Autodesk Inventor part; units mm, degrees
ref_plane "YZ Plane" through (0, 0, 0) normal (1, 0, 0) x (0, 1, 0)
ref_plane "XZ Plane" through (0, 0, 0) normal (0, 1, 0) x (-1, 0, 0)
ref_plane "XY Plane" through (0, 0, 0) normal (0, 0, 1) x (1, 0, 0)
sketch "Sketch1" plane through (0, 0, 0) normal (0, 0, 1) x (1, 0, 0)
  line L0 (0, 0) -> (3294.2276, 1099.144)
  line L1 (3294.2276, 1246.4151) -> (-135.0962, 102.1952)
  line L2 (0, 0) -> (-135.0962, 0)
  line L3 (-135.0962, 0) -> (-135.0962, 102.1952)
  line L4 (-135.0962, 102.1952) -> (1627.6312, 690.3426)
  line L5 (3294.2276, 1099.144) -> (3263.9, 1099.144)
  line L6 (3294.2276, 1099.144) -> (3294.2276, 1246.4151)
  line L7 (-88.9, 0) -> (-88.9, 117.6089)
  line L8 (3263.9, 1089.025) -> (3263.9, 1236.2961)
  line L9 (-135.0962, 102.1952) -> (-160.4962, 102.1952)
  line L10 (-160.4962, 102.1952) -> (-160.4962, 0)
  line L11 (-160.4962, 0) -> (-135.0962, 0)
  line L12 (-135.0962, 102.1952) -> (-140.1208, 117.2541)
  line L13 (-140.1208, 117.2541) -> (150.6173, 214.261)
  line L14 (150.6173, 214.261) -> (155.6418, 199.2021)
  line L15 (-27.6261, 154.7888) -> (-28.631, 157.8005)
  line L16 (-28.631, 157.8005) -> (-173.1962, 109.5652)
  line L17 (-173.1962, 109.5652) -> (-163.6712, 101.107)
  line L18 (-163.6712, 101.107) -> (-163.6712, 92.6488)
  line L19 (-163.6712, 92.6488) -> (-173.1962, 86.9102)
  line L20 (-171.5578, 84.1906) -> (-160.4962, 90.855)
  line L21 (-160.4962, 90.855) -> (-160.4962, 102.5338)
  line L22 (-160.4962, 102.5338) -> (-166.9808, 108.292)
  line L23 (-166.9808, 108.292) -> (-27.6261, 154.7888)
  line L24 (-171.5578, 84.1906) -> (-173.1962, 86.9102)
  line L25 (-173.1962, 109.5652) -> (-173.1962, 86.9102)
  line L26 (3163.3672, 1202.7525) -> (3162.3623, 1205.7643)
  line L27 (3162.3623, 1205.7643) -> (3306.9276, 1253.9996)
  line L28 (3163.3672, 1202.7525) -> (3293.697, 1246.2381)
  line L29 (3293.697, 1246.2381) -> (3294.2276, 1246.7092)
  line L30 (3306.9276, 1253.9996) -> (3297.4026, 1245.5414)
  line L31 (3297.4026, 1245.5414) -> (3297.4026, 1237.0832)
  line L32 (3294.2276, 1246.7092) -> (3294.2276, 1235.2894)
  line L33 (3297.4026, 1237.0832) -> (3306.9276, 1231.3446)
  line L34 (3306.9276, 1231.3446) -> (3305.2891, 1228.625)
  line L35 (3305.2891, 1228.625) -> (3294.2276, 1235.2894)
  line L36 (3306.9276, 1253.9996) -> (3306.9276, 1231.3446)
  point P0 (-160.4962, 90.855)
  point P1 (-160.4962, 101.4128)
  dimension "d5" = 139.7
  dimension "d17" = 88.9
  dimension "d19" = 3352.8
  dimension "d23" = 30.3276
  dimension "d28" = 46.1962
  dimension "d33" = 1089.025
  dimension "d36" = 25.4
  dimension "d37" = 15.875
  dimension "d49" = 3.175
  dimension "d50" = 3.175
  dimension "d51" = 3.175
  dimension "d52" = 3.175
  dimension "d54" = 8.4582
  dimension "d55" = 8.4582
  dimension "d61" = 8.4582
  dimension "d62" = 152.4
  dimension "d63" = 3.175
  dimension "d65" = 12.7
  dimension "d73" = 152.4
  dimension "d74" = 12.7
  dimension "d75" = 3.175
  dimension "d76" = 3.175
  dimension "d78" = 8.4582
  dimension "d79" = 8.4582
  dimension "d80" = 8.4582
extrude "Extrusion2" add sketch "Sketch1" along normal blind 2485.0598 contours L6 L32 L29 L1 L26 L27 L30 L31 L33 L34 L35
properties part number "Drip_Edge_For_Front_With_Length_97.504_Inches" material "Aluminum 6061"
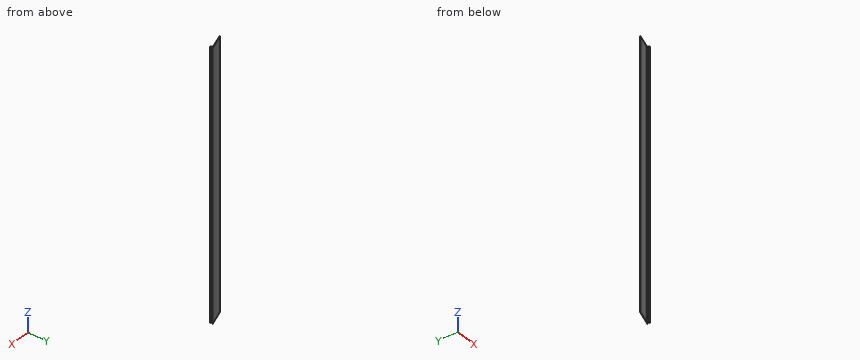
The listing builds one solid part. Answer for the finished solid, in the listing's coordinates (mm). Coordinates: 2 decimals unless noted, no trailing zeros. Loops run counter-clockwise (first coordinate to the right, second up) from the corner with the lowest first, then second, coordinate; pieces in that order, holes last.
1) Flat-ended cylindrical pins translate along their axes: pin 1 Ø1.5 at (x, z) = (3274.5, 2192) entering from -Y; pin 2 Ø8 at (x, y) = (3265.5, 1230) entering from -Z; pin 3 Ø12 at (x, z) = (3240.5, 1350) entering from +Y; pin 4 Ø1.5 at (x, z) = (3207.5, 883) entering from -Y. Find the tip coordinate at first contact, or state that the pin passes through.
2) Find section C-C on y = 1218.5. Write down the section's boundary in (x, z), then the cut area to 3 significant figures.
3) Find the intervals of material crossed by L1, parallel to Y at x = 3233, z = 723.5; L2, parallel to Y at x = 3265, z = 179, in increasing order.
4) Find section B-B on x = 3205.5. Write down the section's boundary in (y, z), then the cut area to 3 significant figures.
5) Find section A-A on z = 323.5. Write down the section's boundary in (x, y) (1 decimal).
Values:
1. pin 1: stops at y = 1239.58
1. pin 2: passes through
1. pin 3: stops at y = 1233.84
1. pin 4: stops at y = 1217.23
2. outline: (3200.53, 0) - (3210.56, 0) - (3210.56, 2485.06) - (3200.53, 2485.06) - close
2. area: 24,900 mm2
3. L1: y = 1225.99 to 1229.33
3. L2: y = 1236.66 to 1240.01
4. outline: (1216.81, 0) - (1220.16, 0) - (1220.16, 2485.06) - (1216.81, 2485.06) - close
4. area: 8,320 mm2
5. outline: (3162.4, 1205.8) - (3163.4, 1202.8) - (3293.7, 1246.2) - (3294.2, 1246.7) - (3294.2, 1235.3) - (3305.3, 1228.6) - (3306.9, 1231.3) - (3297.4, 1237.1) - (3297.4, 1245.5) - (3306.9, 1254) - close
